Input: dimensioned drawing with shaded views. Units: mm. Origin: part minimum x, y, z. Give positions to 0.01 mm unless a question says otherwise; leave off trailing zeros. Write each loop counter-clockwise with the first axis right and the second up, starting at its lowest first coordinate (ties: lowest second). Pieces come first, ordered by that corner, then holes.
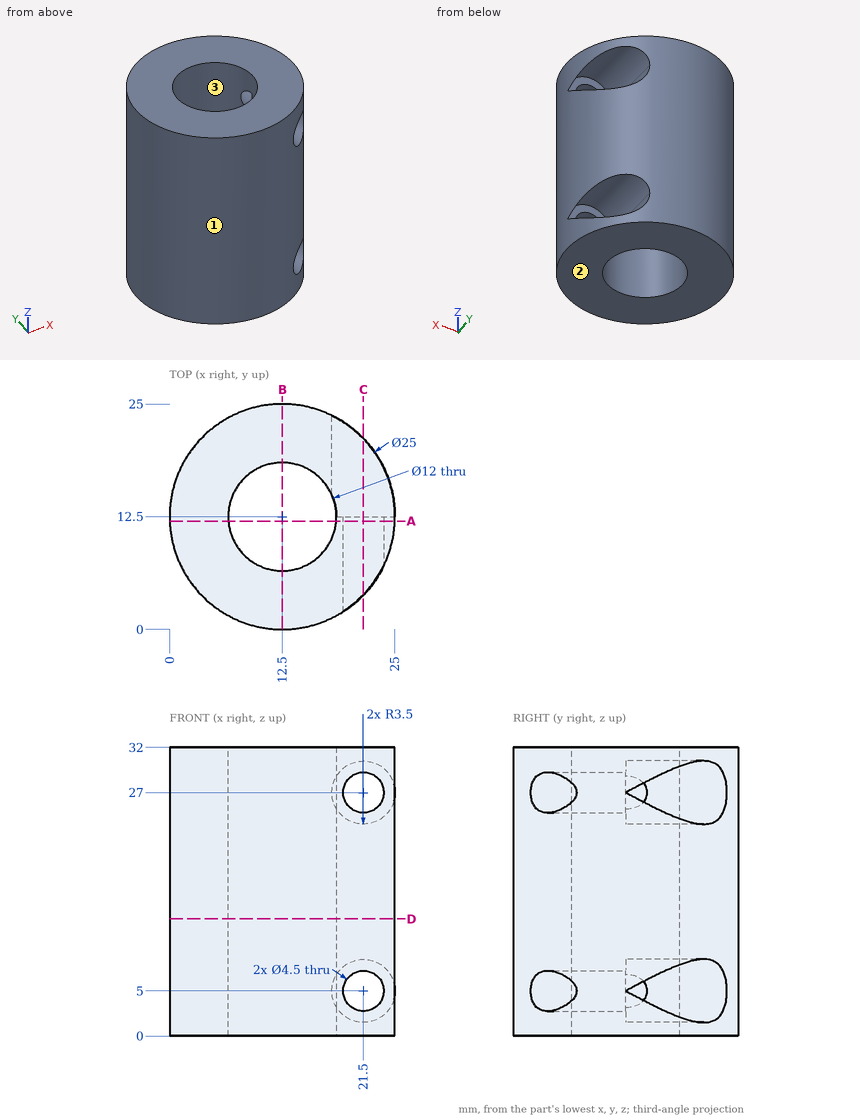
Item 1: Section B-B (x = 12.5). Return loops of the section in (y, z), and give its area (3 significant figures).
Item 2: Section D-D (z = 13). Return loops of the section in (x, y), and give its area (3 significant figures).
Item 3: Mould query, pull axis X, two halves, no side actions, for the marked faces 1, 2 and 3. Classes: +X half, -X half, draft (parallel to the pull), parting line (faces both ways), or undercut.
Item 4: Section C-C (x = 21.5). Return loops of the section in (y, z), and give its area (3 significant figures).
Item 5: Ray query, line 1 (Z direction, x = 21.5, y = 6.75); line 2 (Z direction, x = 21.75, y = 17.5); line 3 (X direction, y = 14, z = 24). Return the intervals inside material, ascending.
Item 6: Section A-A (y = 12). Return loops of the section in (x, z), and give its area (3 significant figures).
Item 7: Pin query (flat end, axial travel): pin 1 (9.5 mm diameter, centred on x = 12.5, y = 12.5, fed in from -Z); pin 2 (8 mm diameter, centred on x = 19.5, z = 14, fed in from +Y); pin 3 (2 mm diameter, centred on x = 17.5, z = 15.5, fed in from -Y); pin 4 (5 mm diameter, centred on x = 21.5, z = 27, fed in from +Y). Return the tip coordinate at first contact, or that it passes through.
Solved:
1. outline: (0, 0) - (6.5, 0) - (6.5, 32) - (0, 32) - close; (18.5, 0) - (25, 0) - (25, 32) - (18.5, 32) - close
1. area: 416 mm2
2. outline: circle Ø25 at (12.5, 12.5); hole circle Ø12 at (12.5, 12.5)
2. area: 378 mm2
3. face 1: parting line
3. face 2: draft
3. face 3: undercut
4. outline: (3.83, 0) - (21.17, 0) - (21.17, 1.5) - (12.5, 1.5) - (12.5, 2.75) - (3.83, 2.75) - close; (3.83, 7.25) - (12.5, 7.25) - (12.5, 8.5) - (21.17, 8.5) - (21.17, 23.5) - (12.5, 23.5) - (12.5, 24.75) - (3.83, 24.75) - close; (3.83, 29.25) - (12.5, 29.25) - (12.5, 30.5) - (21.17, 30.5) - (21.17, 32) - (3.83, 32) - close
4. area: 356 mm2
5. line 1: z = 0 to 2.75, 7.25 to 24.75, 29.25 to 32
5. line 2: z = 0 to 1.51, 8.49 to 23.51, 30.49 to 32
5. line 3: x = 0.09 to 6.69, 18.31 to 19.7, 23.3 to 24.91
6. outline: (0.01, 0) - (6.52, 0) - (6.52, 32) - (0.01, 32) - close; (18.48, 0) - (24.99, 0) - (24.99, 32) - (18.48, 32) - close; hole circle Ø4.5 at (21.5, 5); hole circle Ø4.5 at (21.5, 27)
6. area: 385 mm2
7. pin 1: passes through
7. pin 2: stops at y = 24.63
7. pin 3: stops at y = 0.66
7. pin 4: stops at y = 12.5
